```python
from build123d import *

# Parameters (mm, degrees)
SKETCH1_R           = 1.6
SKETCH1_R_2         = 2.1
BOSS_EXTRUDE1_DEPTH = 3
CUT_EXTRUDE1_DEPTH  = 4
FILLET1_R           = 3


with BuildPart() as part:
    # Sketch1 → Boss-Extrude1 (new body)
    with BuildSketch(Plane(origin=(0, 0, 0), x_dir=(1, 0, 0), z_dir=(0, 1, 0))):
        Polygon((0, 0), (0, 12), (15, -3), (75, -3), (90, 12), (90, 0), (75, -15), (15, -15), align=None)
        with Locations((7.5, -1.5)):
            Circle(SKETCH1_R, mode=Mode.SUBTRACT)
        with Locations((37.5, -9)):
            Circle(SKETCH1_R_2, mode=Mode.SUBTRACT)
        with Locations((82.5, -1.5)):
            Circle(SKETCH1_R, mode=Mode.SUBTRACT)
        with Locations((52.5, -9)):
            Circle(SKETCH1_R_2, mode=Mode.SUBTRACT)
    extrude(amount=BOSS_EXTRUDE1_DEPTH)

    # Sketch2 → Cut-Extrude1 (cut, through all)
    with BuildSketch(Plane(origin=(0, 3, 0), x_dir=(1, 0, 0), z_dir=(0, 1, 0))):
        Polygon((15, -3), (17.9, -5.9), (72.1, -5.9), (75, -3), align=None)
        Polygon((12.1, -12.1), (77.9, -12.1), (75, -15), (15, -15), align=None)
    extrude(amount=-CUT_EXTRUDE1_DEPTH, mode=Mode.SUBTRACT)

    # Fillet1
    fillet1_edges = [part.edges().sort_by_distance(p)[0] for p in [
        (0, 1.5, 0),
        (0, 1.5, -12),
        (90, 1.5, -12),
        (90, 1.5, 0),
        (72.1, 1.5, 5.9),
        (17.9, 1.5, 5.9),
        (12.1, 1.5, 12.1),
        (77.9, 1.5, 12.1),
    ]]
    fillet(fillet1_edges, radius=FILLET1_R)


solid = part.part
```
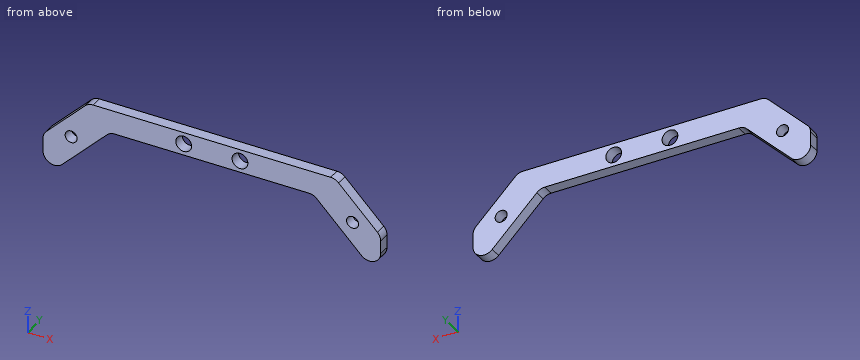
Geometry: final body of the model. Coordinates: model frame, mm. Coordinates: 2 decimals unless noted, no trailing zeros. Write each loop counter-clockwise with the first axis right and the second up, starting at its lowest first coordinate (ties: lowest second). Pieces come first, ordered by that corner, then holes. Notation, with made-up numbers: M 22.25,-2.5 L 27.25,-2.5 A20 ccw 27.25,33.5 Z; hole C 51.5,-3 d10. An arc over 180 degrees is marked long. Use CSV: the item, a comma, the result in double quotes. Start each with the question number.
1. Cut plane A-A on x = 37.5. Return the cut outline in (y, z).
2. Cut plane D-D on z = 4. Return the cut outline in (x, y), plus the area to 3 significant figures.
3. Ray query, probe 1 along X at (y, z) = (1.5, 1.5); probe 2 along X at (y, z) = (1.35, 9.25); probe 3 along Z at (x, y) = (37.5, 1.3). Return the intervals inside material, ascending.
4. First-contact query: P1, Ø2.5, axis at x = 7.5, z = 1.5, coming from the -Y side; P2, Ø1.5, axis at x = 49.5, y = 1.5, coming from the -Z side. Flat tips, straight axial feed; report the tip coordinate or a pass-through.
5. Cut plane B-B on z = 9. Return the cut outline in (x, y).
6. Cut plane C-C on y = 0.8. Return the cut outline in (x, z).
Entries:
1,outline,"M 0,5.9 L 3,5.9 L 3,6.9 L 0,6.9 Z; M 0,11.1 L 3,11.1 L 3,12.1 L 0,12.1 Z"
2,outline,"M 4,0 L 16,0 L 16,3 L 4,3 Z; M 74,0 L 86,0 L 86,3 L 74,3 Z"
2,area,"72.0 mm²"
3,probe 1,"1.5 to 5.9, 9.1 to 13.5, 76.5 to 80.9, 84.1 to 88.5"
3,probe 2,"9.25 to 35.41, 39.59 to 50.41, 54.59 to 80.75"
3,probe 3,"5.9 to 6.9, 11.1 to 12.1"
4,P1,"through"
4,P2,"z = 5.9"
5,outline,"M 9,0 L 35.4,0 L 35.4,3 L 9,3 Z; M 39.6,0 L 50.4,0 L 50.4,3 L 39.6,3 Z; M 54.6,0 L 81,0 L 81,3 L 54.6,3 Z"
6,outline,"M 0,-4.76 A3 ccw 5.12,-6.88 L 17.02,5.02 A3 cw 19.14,5.9 L 70.86,5.9 A3 cw 72.98,5.02 L 84.88,-6.88 A3 ccw 90,-4.76 L 90,-1.24 A3 ccw 89.12,0.88 L 78.78,11.22 A3 ccw 76.66,12.1 L 13.34,12.1 A3 ccw 11.22,11.22 L 0.88,0.88 A3 ccw 0,-1.24 Z; hole C 7.5,1.5 d3.2; hole C 37.5,9 d4.2; hole C 52.5,9 d4.2; hole C 82.5,1.5 d3.2"
